Design review of the part built by this model. Coordinates are the model's own, in mm. A direction names the side the tool comes from. Coordinates: 2 decimals unless noted, no trailing zeros. Loops run counter-clockwise (first coordinate to the right, second up) from the corner with the lowest first, then second, coordinate; pieces in that order, holes last. Notation, with made-up numbers: (6, -20) - (32, -20) arc R11 ccw to (32, -13) - close; hole circle Ø1 at (57, 74.5). An arc over 180 degrees is marked (long way). Return JSON: item names as keys, results as strings. Group by question number.
Autodesk Inventor part; units mm, degrees
ref_plane "YZ Plane" through (0, 0, 0) normal (1, 0, 0) x (0, 1, 0)
ref_plane "XZ Plane" through (0, 0, 0) normal (0, 1, 0) x (-1, 0, 0)
ref_plane "XY Plane" through (0, 0, 0) normal (0, 0, 1) x (1, 0, 0)
sketch "Sketch1" plane through (0, 0, 0) normal (0, 1, 0) x (-1, 0, 0)
  line L0 (0, -7.3323) -> (-6.35, -3.6662)
  line L1 (-6.35, -3.6662) -> (-6.35, 3.6662)
  line L2 (-6.35, 3.6662) -> (0, 7.3323)
  line L3 (0, 7.3323) -> (6.35, 3.6662)
  line L4 (6.35, 3.6662) -> (6.35, -3.6662)
  line L5 (6.35, -3.6662) -> (0, -7.3323)
  point P0 (0, 0)
  point P1 (0, 0)
  dimension "d0" = 12.7
extrude "Extrusion1" add sketch "Sketch1" along normal blind 43.18
sketch "Sketch2" plane through (0, 43.18, 0) normal (0, 1, 0) x (1, 0, 0)
  point P0 (0, 0)
  point P1 (0, 0)
hole "Hole1" at (0, 43.18, 0) direction (0, -1, 0) diameter 4.0386 depth 6.35
sketch "Sketch3" plane through (0, 0, 0) normal (0, -1, 0) x (1, 0, 0)
  point P0 (0, 0)
  point P1 (0, 0)
hole "Hole2" at (0, 0, 0) direction (0, 1, 0) diameter 4.0386 depth 6.35
thread "Thread1"
properties part number "Gearboxes_002_Hexshaft my fav" material "Aluminum 6061"
Item 1: Add section A-A (y = 38.5). State the section outline as (x, z) points, then the cut area to 3 significant figures.
Item 2: Add section B-B (z = 0). State the section outline as (x, y) points.
Item 3: Draft analysis for pull direction X (two halves, no side actions). For faces 1 (the face through (6.35, 21, 0)), 2 (the face through (-3.219, 21.288, -5.474)), 3 (the face through (2, 0, -2)), 4 (the face through (-0.607, 3.219, -1.926)), state which applies: pulls with the +X half, pulls with the -X half, needs draft (parallel to the pull), parting line crosses it, or undercut.
Item 4: Add section D-D (y = 16). State the section outline as (x, z) points.
Item 5: Add section C-C (x = -0.5). State the section outline as (y, z) points.
Item 6: For faces 5 (the face through (0, 36.83, 0)), 6 (the face through (-6.35, 21, 0)), 7 (the face through (0, 6.35, 0)), list the 3-axis set-ups (+Z, -Z, +X, -X, +Y, -Y) from which the entire face can be reached by the end or side of a thin tool; tool diameter is ignored.
Item 7: To check wall thickness, follow line 1 (X direction, y = 3.25, z = 0); line 2 (Z direction, x = 0, y = 41.75); line 3 (Z direction, x = 0.75, y = 37.5). State the ranges of each line that lie inside material, in increasing order. Write a range as from..to.
Item 8: For P1, Ø3, axis at x = -2, y = 5.5, coming from the +Z side; P2, Ø4, axis at x = 2.5, z = 0.5, coming from the -Y side; P3, Ø5, axis at x = -3, y = 7, coming from the -Z side; P4, Ø3, axis at x = 0, z = 0, coming from the -Y side, all flat-tipped, find the tip position at first contact; note any pin that passes through.
Answers below:
{
 "1": {"outline": "(-6.35, -3.67) - (0, -7.33) - (6.35, -3.67) - (6.35, 3.67) - (0, 7.33) - (-6.35, 3.67) - close; hole circle Ø4.04 at (0, 0)", "area": "127 mm^2"},
 "2": {"outline": "(-6.35, 0) - (-2.02, 0) - (-2.02, 6.35) - (2.02, 6.35) - (2.02, 0) - (6.35, 0) - (6.35, 43.18) - (2.02, 43.18) - (2.02, 36.83) - (-2.02, 36.83) - (-2.02, 43.18) - (-6.35, 43.18) - close"},
 "3": {"face 1": "pulls with the +X half", "face 2": "pulls with the -X half", "face 3": "needs draft", "face 4": "undercut"},
 "4": {"outline": "(-6.35, -3.67) - (0, -7.33) - (6.35, -3.67) - (6.35, 3.67) - (0, 7.33) - (-6.35, 3.67) - close"},
 "5": {"outline": "(0, -7.04) - (43.18, -7.04) - (43.18, -1.96) - (36.83, -1.96) - (36.83, 1.96) - (43.18, 1.96) - (43.18, 7.04) - (0, 7.04) - (0, 1.96) - (6.35, 1.96) - (6.35, -1.96) - (0, -1.96) - close"},
 "6": {"face 5": "+Y", "face 6": "+Z, -Z, -X, +Y, -Y", "face 7": "-Y"},
 "7": {"line 1": "x = -6.35..-2.02, 2.02..6.35", "line 2": "z = -7.33..-2.02, 2.02..7.33", "line 3": "z = -6.9..-1.87, 1.87..6.9"},
 "8": {"P1": "stops at z = 7.04", "P2": "stops at y = 0", "P3": "stops at z = -7.04", "P4": "stops at y = 6.35"}
}
